Could you check a few things on this model? Use its own coordinates, in mm. A direction names the side the tool comes from. Coordinates: 2 decimals unless noted, no trailing zeros. Loops run counter-clockwise (first coordinate to the right, second up) from the corner with the lowest first, then second, coordinate; pieces in that order, holes last.
1) Imagine slicing it at D-D on x = -12. Please give me the cut outline in (y, z).
2) Imagine slicing it at C-C on y = 1.25. Please give me the cut outline in (x, z).
3) Imagine slicing it at B-B on x = 0. Please give me the cut outline in (y, z).
4) Will these pins go through, and if not, where does the flat tip stop? P1, Ø1.5, axis at x = -2, y = -3, coming from the +Z side; P2, Ø7.5, axis at x = 9.5, z = 4, coming from the +Y side; P3, Ø4, axis at y = 1, z = 1.5, coming from the +X side; P4, Ø5.5, axis at x = -10, z = -5.5, coming from the +Y side.
5) If I drill on line 1 along Z through (x, y) = (-12, -4.25); line 2 along Z through (x, y) = (13.5, -6); line 3 along Y through (x, z) = (0, -10.75), over which ranges is the centre line in solid material (lowest first)?
6) Thinking about a two-plate mould opening in Z: for faces 4 (the face through (0, -5, -15)), 5 (the face through (-17, -8, 0)), 6 (the face through (-10.34, -2.62, 6.48)), which applies, released by +Z, released by -Z, zero draft, split by the parting line, or undercut?
7) Imagine slicing it at A-A on z = 8. Please give me the cut outline in (x, y), plus the area to 3 significant figures.
8) For faces 1 (the face through (-11, 6, 0)), 2 (the face through (12, -11, 0)), 3 (the face through (11, 6, 0)), which set-ups out of +Z, -Z, +X, -X, +Y, -Y let a thin tool reach every point of the face, with its end or its side?
```python
from build123d import *

# Parameters (mm, degrees)
ESQUISSE1_R             = 4
BOSS_EXTRU_1_DEPTH      = 15
BOSS_EXTRU_1_DEPTH_BACK = 15
D_GAGEMENT_M41_D        = 4.5


with BuildPart() as part:
    # Esquisse1 → Boss.-Extru.1 (new body, two sides)
    with BuildSketch(Plane.XY) as boss_extru_1_sk:
        Polygon((-17, -11), (-6.5, -11), (-6, -10.5), (6, -10.5), (6.5, -11), (17, -11), (17, -5), (16, -4), (16, 4.5), (14.5, 6), (7.5, 6), (3.5, 10), (-3.5, 10), (-7.5, 6), (-14.5, 6), (-16, 4.5), (-16, -4), (-17, -5), align=None)
        Circle(ESQUISSE1_R, mode=Mode.SUBTRACT)
    extrude(amount=BOSS_EXTRU_1_DEPTH)
    extrude(boss_extru_1_sk.sketch, amount=-BOSS_EXTRU_1_DEPTH_BACK)

    # D_gagement M41 (through all)
    with Locations(Plane(origin=(0, 6, 0), x_dir=(1, 0, 0), z_dir=(0, 1, 0))):
        with Locations((-12, 8), (12, 8), (12, -8), (-12, -8)):
            Hole(D_GAGEMENT_M41_D / 2)


solid = part.part
```
Filled in:
1. outline: (-11, -15) - (6, -15) - (6, -10.25) - (-11, -10.25) - close; (-11, -5.75) - (6, -5.75) - (6, 5.75) - (-11, 5.75) - close; (-11, 10.25) - (6, 10.25) - (6, 15) - (-11, 15) - close
2. outline: (-16, -15) - (-3.8, -15) - (-3.8, 15) - (-16, 15) - close; (3.8, -15) - (16, -15) - (16, 15) - (3.8, 15) - close; hole circle Ø4.5 at (-12, -8); hole circle Ø4.5 at (-12, 8); hole circle Ø4.5 at (12, -8); hole circle Ø4.5 at (12, 8)
3. outline: (-10.5, -15) - (-4, -15) - (-4, 15) - (-10.5, 15) - close; (4, -15) - (10, -15) - (10, 15) - (4, 15) - close
4. P1: stops at z = 15
4. P2: stops at y = 7.75
4. P3: stops at x = 16
4. P4: stops at y = 6.25
5. line 1: z = -15 to -10.25, -5.75 to 5.75, 10.25 to 15
5. line 2: z = -15 to -9.68, -6.32 to 6.32, 9.68 to 15
5. line 3: y = -10.5 to -4, 4 to 10
6. face 4: released by -Z
6. face 5: zero draft
6. face 6: undercut
7. outline: (-17, -11) - (-14.25, -11) - (-14.25, 6) - (-14.5, 6) - (-16, 4.5) - (-16, -4) - (-17, -5) - close; (-9.75, -11) - (-6.5, -11) - (-6, -10.5) - (6, -10.5) - (6.5, -11) - (9.75, -11) - (9.75, 6) - (7.5, 6) - (3.5, 10) - (-3.5, 10) - (-7.5, 6) - (-9.75, 6) - close; (14.25, -11) - (17, -11) - (17, -5) - (16, -4) - (16, 4.5) - (14.5, 6) - (14.25, 6) - close; hole circle Ø8 at (0, 0)
7. area: 389 mm2
8. face 1: +Z, -Z, -X, +Y
8. face 2: +Z, -Z, +X, -X, -Y
8. face 3: +Z, -Z, +X, +Y
